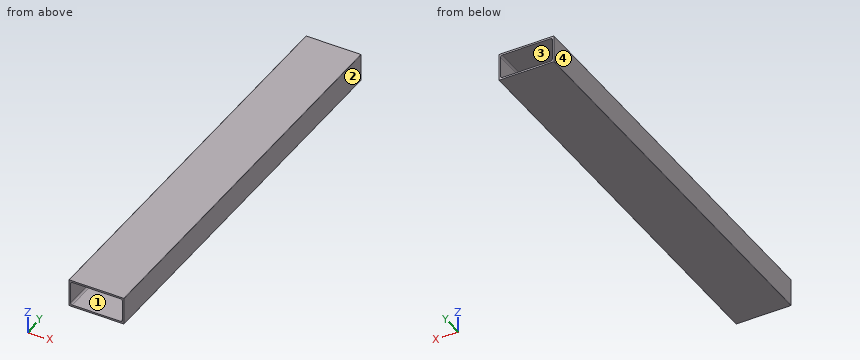
```python
from build123d import *

# Parameters (mm, degrees)
F0_W     = 50.8
F0_H     = 25.4
F1_DEPTH = 381
F2_W     = 47.6504
F2_H     = 22.2504
F3_DEPTH = 381
F4_R     = 1.524
F5_R     = 0.254


with BuildPart() as f1:
    # F0 (on Front) → F1 (new body)
    with BuildSketch(Plane.XZ):
        Rectangle(F0_W, F0_H)
    extrude(amount=F1_DEPTH)

    # F2 (on face) → F3 (cut, through all)
    with BuildSketch(Plane.XZ.offset(381)):
        Rectangle(F2_W, F2_H)
    extrude(amount=-F3_DEPTH, mode=Mode.SUBTRACT)

    # F4
    f4_edges = [f1.edges().sort_by_distance(p)[0] for p in [
        (23.8252, -190.5, -11.1252),
        (23.8252, -190.5, 11.1252),
        (-23.8252, -190.5, -11.1252),
        (-23.8252, -190.5, 11.1252),
    ]]
    fillet(f4_edges, radius=F4_R)

    # F5
    f5_edges = [f1.edges().sort_by_distance(p)[0] for p in [
        (-25.4, -190.5, 12.7),
        (25.4, -190.5, 12.7),
        (25.4, -190.5, -12.7),
        (-25.4, -190.5, -12.7),
    ]]
    fillet(f5_edges, radius=F5_R)


solid = f1.part
```
Input: part model. Units: mm. Frame: model coordinates. Face numbers are marked on the shaded views. Round coordinates to 2 decimals unless told otherwise and drop trailing zeros. Loops run counter-clockwise (first coordinate to the right, second up) from the corner with the lowest first, then second, coordinate; pieces in that order, holes last.
1) Material intervals for line 1 (X direction, y = -254.5, z = 4); line 2 (Z direction, x = -19, y = -341); line 3 (X direction, y = -38, z = 10.5), sorted ascending.
Ans:
line 1: x = -25.4 to -23.83, 23.83 to 25.4
line 2: z = -12.7 to -11.13, 11.13 to 12.7
line 3: x = -25.4 to -23.53, 23.53 to 25.4
2) Section query B-B on x = 6. Return the cut outline in (y, z), plus the area to 3 significant figures.
Ans:
outline: (-381, -12.7) - (0, -12.7) - (0, -11.13) - (-381, -11.13) - close; (-381, 11.13) - (0, 11.13) - (0, 12.7) - (-381, 12.7) - close
area: 1,200 mm2
3) Pull-direction query (X, two-part tool) for the marked faces 1, 2, 3 and 4; classes: released by +X, released by -X, zero draft, split by the parting line, or undercut.
Ans:
face 1: undercut
face 2: released by +X
face 3: undercut
face 4: released by -X
4) Section query A-A on y = -208. Return the cut outline in (x, z), plus the area to 3 significant figures.
Ans:
outline: (-25.4, -12.45) arc R0.25 ccw to (-25.15, -12.7) - (25.15, -12.7) arc R0.25 ccw to (25.4, -12.45) - (25.4, 12.45) arc R0.25 ccw to (25.15, 12.7) - (-25.15, 12.7) arc R0.25 ccw to (-25.4, 12.45) - close; hole (-23.83, -9.6) arc R1.52 ccw to (-22.3, -11.13) - (22.3, -11.13) arc R1.52 ccw to (23.83, -9.6) - (23.83, 9.6) arc R1.52 ccw to (22.3, 11.13) - (-22.3, 11.13) arc R1.52 ccw to (-23.83, 9.6) - close
area: 232 mm2
5) Section query C-C on z = 3.5. Return the cut outline in (x, y), plus the area to 3 significant figures.
Ans:
outline: (-25.4, -381) - (-23.83, -381) - (-23.83, 0) - (-25.4, 0) - close; (23.83, -381) - (25.4, -381) - (25.4, 0) - (23.83, 0) - close
area: 1,200 mm2
